```python
from build123d import *

# Parameters (mm, degrees)
SKETCH1_R           = 26
BOSS_EXTRUDE1_DEPTH = 8
SKETCH2_R           = 6.1
CUT_EXTRUDE2_DEPTH  = 3
SKETCH1_11_R        = 3.82
BOSS_EXTRUDE3_DEPTH = 9
FILLET1_R           = 2.5
SKETCH3_R           = 1.15
SKETCH3_R_2         = 1.160199873
CUT_EXTRUDE3_DEPTH  = 6
CHAMFER1_SIZE       = 0.5


with BuildPart() as part:
    # Sketch1 → Boss-Extrude1 (new body)
    with BuildSketch(Plane(origin=(0, 0, 0), x_dir=(1, 0, 0), z_dir=(0, 1, 0))):
        Circle(SKETCH1_R)
    extrude(amount=BOSS_EXTRUDE1_DEPTH)

    # Sketch2 → Cut-Extrude2 (cut)
    with BuildSketch(Plane.XZ):
        Circle(SKETCH2_R)
    extrude(amount=-CUT_EXTRUDE2_DEPTH, mode=Mode.SUBTRACT)

    # Sketch1<11> → Boss-Extrude3 (add)
    with BuildSketch(Plane(origin=(0, 0, 0), x_dir=(1, 0, 0), z_dir=(0, 1, 0))):
        with Locations((-13.647160877, 13.647160877)):
            Circle(SKETCH1_11_R)
        with Locations((0, 19.3)):
            Circle(SKETCH1_11_R)
        with Locations((13.647160877, 13.647160877)):
            Circle(SKETCH1_11_R)
        with Locations((19.3, 0)):
            Circle(SKETCH1_11_R)
        with Locations((13.647160877, -13.647160877)):
            Circle(SKETCH1_11_R)
        with Locations((0, -19.3)):
            Circle(SKETCH1_11_R)
        with Locations((-13.647160877, -13.647160877)):
            Circle(SKETCH1_11_R)
        with Locations((-19.3, 0)):
            Circle(SKETCH1_11_R)
    extrude(amount=-BOSS_EXTRUDE3_DEPTH)

    # Fillet1
    fillet1_edges = [part.edges().sort_by_distance(p)[0] for p in [
        (-26, 0, 0),
        (-26, 8, 0),
    ]]
    fillet(fillet1_edges, radius=FILLET1_R)

    # Sketch3 → Cut-Extrude3 (cut)
    with BuildSketch(Plane(origin=(0, 8, 0), x_dir=(1, 0, 0), z_dir=(0, 1, 0))):
        with Locations((-8, 16)):
            Circle(SKETCH3_R)
        with Locations((8, 16)):
            Circle(SKETCH3_R)
        with Locations((-8, 8)):
            Circle(SKETCH3_R)
        with Locations((8, 8)):
            Circle(SKETCH3_R)
        with Locations((-8, -8)):
            Circle(SKETCH3_R)
        with Locations((8, -8)):
            Circle(SKETCH3_R)
        with Locations((-8, -16)):
            Circle(SKETCH3_R)
        with Locations((8, -16)):
            Circle(SKETCH3_R)
        with Locations((-8, 0)):
            Circle(SKETCH3_R)
        with Locations((8, 0)):
            Circle(SKETCH3_R_2)
    extrude(amount=-CUT_EXTRUDE3_DEPTH, mode=Mode.SUBTRACT)

    # Chamfer1
    chamfer1_edges = [part.edges().sort_by_distance(p)[0] for p in [
        (-17.467160877, -9, -13.647160877),
        (-3.82, -9, -19.3),
        (9.827160877, -9, -13.647160877),
        (15.48, -9, 0),
        (9.827160877, -9, 13.647160877),
        (-3.82, -9, 19.3),
        (-17.467160877, -9, 13.647160877),
        (-23.12, -9, 0),
    ]]
    chamfer(chamfer1_edges, length=CHAMFER1_SIZE)


solid = part.part
```
The listing builds one solid part. Answer for the finished solid, in the listing's coordinates (mm). A direction names the side the tool comes from. Coordinates: 2 decimals unless noted, no trailing zeros. Loops run counter-clockwise (first coordinate to the right, second up) from the corner with the lowest first, then second, coordinate; pieces in that order, holes last. Notation, with made-up numbers: (87, -16) - (140, -16) arc R28 cw to (140, 3) - close; hole circle Ø10 at (61.25, -8). An arc over 180 degrees is marked (long way). Write item = value, one per line.
1) Section B-B (y = 1.25) is taken. Determine the outline of the cut face in (x, z), plus the area to 3 significant figures.
Responses:
outline = circle Ø51.33 at (0, 0); hole circle Ø12.2 at (0, 0)
area = 1,950 mm^2
2) Section A-A (y = -7.25) is taken. Determine the outline of the cut face in (x, z).
Responses:
outline = circle Ø7.64 at (-19.3, 0); circle Ø7.64 at (-13.65, -13.65); circle Ø7.64 at (-13.65, 13.65); circle Ø7.64 at (0, -19.3); circle Ø7.64 at (0, 19.3); circle Ø7.64 at (13.65, -13.65); circle Ø7.64 at (13.65, 13.65); circle Ø7.64 at (19.3, 0)
3) Determine the mould class of faces 3 (the face through (0, 3, 0)), 4 (the face through (0, 8, 0)) for opening direction X: pulls with the +X half, pulls with the -X half, needs draft (parallel to the pull), parting line crosses it, or undercut.
Responses:
face_3 = undercut
face_4 = needs draft
4) Each of these flat-tipped pins is pushed along its axis until it touches: P1, Ø3, axis at y = 0, z = -12.5, coming from the +X side; P2, Ø0.7, axis at x = -8, z = 0, coming from the +Y side; P3, Ø4, axis at y = 3, z = -15.5, coming from the -X side. Where does it stop, or does it pass through?
Responses:
P1 = 22.86
P2 = 2
P3 = -22.22
5) Which of the six approach directions +Z, -Z, +X, -X, +Y, -Y give full straight-line access (tool end or side, diameter ignored) to faces 1 (the face through (-6.938, 5.042, 8.44)), 2 (the face through (17.176, -4.19, 15.11))?
Responses:
face_1 = +Y
face_2 = -Y
6) Find the intervals of material crossed by line 1 along X through (y, z) = (3.65, 0); line 2 along Z through (x, y) = (-16, -3.75); line 3 along Z through (x, y) = (8, 6.75), in increasing order.
Responses:
line_1 = -26 to -9.15, -6.85 to 6.84, 9.16 to 26
line_2 = -16.66 to -10.64, -1.92 to 1.92, 10.64 to 16.66
line_3 = -24.39 to -17.15, -14.85 to -9.15, -6.85 to -1.16, 1.16 to 6.85, 9.15 to 14.85, 17.15 to 24.39
